from build123d import *

# Parameters (mm, degrees)
CROQUIS1_R                     = 9.525
SALIENTE_EXTRUIR1_DEPTH        = 101.6
CROQUIS2_W                     = 19.05
CROQUIS2_H                     = 20.32
CORTAR_EXTRUIR1_DEPTH          = 12.7
CORTAR_EXTRUIR2_DEPTH          = 12.7
TALADRO_ROSCADO_5_16_181_D     = 6.5278
TALADRO_ROSCADO_5_16_181_DEPTH = 22.9235
TALADRO_ROSCADO_5_16_181_TIP   = 1.961148974
TALADRO_ROSCADO_5_16_182_D     = 6.5278
TALADRO_ROSCADO_5_16_182_DEPTH = 19.7485
TALADRO_ROSCADO_5_16_182_TIP   = 1.961148974


with BuildPart() as part:
    # Croquis1 → Saliente-Extruir1 (new, symmetric)
    with BuildSketch(Plane(origin=(0, 0, 0), x_dir=(1, 0, 0), z_dir=(0, 1, 0))):
        with Locations(Location((0, 0, 0), (0, 0, 270))):
            Circle(CROQUIS1_R)
    extrude(amount=SALIENTE_EXTRUIR1_DEPTH, both=True)

    # Croquis2 → Cortar-Extruir1 (cut)
    with BuildSketch(Plane(origin=(0, 0, 0), x_dir=(0, 0, -1), z_dir=(1, 0, 0))):
        with Locations((0, -91.44)):
            Rectangle(CROQUIS2_W, CROQUIS2_H)
    extrude(amount=-CORTAR_EXTRUIR1_DEPTH, mode=Mode.SUBTRACT)

    # Croquis3 → Cortar-Extruir2 (cut)
    with BuildSketch(Plane.ZY):
        with BuildLine():
            ThreePointArc((0, -101.6), (-6.735192091, -98.810192091), (-9.525, -92.075))
            Line((-9.525, -92.075), (-9.525, -101.6))
            Line((-9.525, -101.6), (0, -101.6))
        make_face()
        with BuildLine():
            ThreePointArc((9.525, -92.075), (6.735192091, -98.810192091), (0, -101.6))
            Line((0, -101.6), (9.525, -101.6))
            Line((9.525, -101.6), (9.525, -92.075))
        make_face()
    extrude(amount=-CORTAR_EXTRUIR2_DEPTH, mode=Mode.SUBTRACT)

    # Taladro roscado 5/16-181
    with Locations(Plane.ZY):
        with Locations((0, -92.075)):
            Hole(TALADRO_ROSCADO_5_16_181_D / 2, depth=TALADRO_ROSCADO_5_16_181_DEPTH)
            with Locations((0, 0, -(TALADRO_ROSCADO_5_16_181_DEPTH + TALADRO_ROSCADO_5_16_181_TIP / 2))):  # 118° drill point
                Cone(0, TALADRO_ROSCADO_5_16_181_D / 2, TALADRO_ROSCADO_5_16_181_TIP, mode=Mode.SUBTRACT)

    # Taladro roscado 5/16-182
    with Locations(Plane(origin=(0, 101.6, 0), x_dir=(1, 0, 0), z_dir=(0, 1, 0))):
        with Locations((0, 0)):
            Hole(TALADRO_ROSCADO_5_16_182_D / 2, depth=TALADRO_ROSCADO_5_16_182_DEPTH)
            with Locations((0, 0, -(TALADRO_ROSCADO_5_16_182_DEPTH + TALADRO_ROSCADO_5_16_182_TIP / 2))):  # 118° drill point
                Cone(0, TALADRO_ROSCADO_5_16_182_D / 2, TALADRO_ROSCADO_5_16_182_TIP, mode=Mode.SUBTRACT)


solid = part.part
Read the model definition and answer for the solid it produces. Units are mm, in the model's axes. A direction names the side the tool comes from. Round coordinates to 2 decimals unless told otherwise and drop trailing zeros. Write each loop counter-clockwise with the first axis right and the second up, starting at its lowest first coordinate (ties: lowest second). Pieces come first, ordered by that corner, then holes.
Q1. A tool of negligible diameter and unlimited length cuts with its end or side. For faces 1 (the face through (4.83, -91.93, 3.26)), 2 (the face through (-4, -81.28, 0)), from which of +Z, -Z, +X, -X, +Y, -Y can it reach the whole face along a straight path? Write none if from no direction.
Values:
face 1: +X, -X
face 2: +Z, -Z, -X, -Y
Q2. Straight lines are drawn through the part: line 1 (Z direction, x = 0, y = 96) (3 decimals); line 2 (Y direction, x = 7.25, z = 0); line 3 (Y direction, x = -3.25, z = 4.25). For each, find the intervals that lie inside material, in ascending order.
Values:
line 1: z = -9.525 to -3.264, 3.264 to 9.525
line 2: y = -101.6 to -95.34, -88.81 to 101.6
line 3: y = -81.28 to 101.6
Q3. Find section A-A on y = -73. Determine the outline of the cut face in (x, z) (3 decimals), and give its area (3 significant figures).
Values:
outline: circle Ø19.05 at (0, 0)
area: 285 mm2
Q4. The mould has two halves that part along Z. Classify faces 3 (the face through (0.708, 91.588, 3.186)), 4 (the face through (9.444, 1.422, -1.24)), 5 (the face through (0, 101.6, 4)): released by +Z, released by -Z, zero draft, split by the parting line, or undercut.
Values:
face 3: undercut
face 4: split by the parting line
face 5: zero draft
Q5. Find section B-B on x = -5. Determine the outline of the cut face in (y, z).
Values:
outline: (-81.28, -8.11) - (101.6, -8.11) - (101.6, 8.11) - (-81.28, 8.11) - close
Q6. Flat-ended cylindrical pins translate along their axes: P1, Ø10, axis at x = -6.5, y = 8.5, coming from the -Z side; P2, Ø5, axis at x = -4.5, z = -4.5, coming from the -Y side; P3, Ø1, axis at y = -51.5, z = -2, coming from the -X side. Find the tip coordinate at first contact, or state that the pin passes through.
Values:
P1: stops at z = -9.41
P2: stops at y = -81.28
P3: stops at x = -9.41
